```python
from build123d import *

# Parameters (mm, degrees)
F0_R     = 2.5
F1_DEPTH = 25
F3_R     = 15
F5_T     = -1


with BuildPart() as f1:
    # F0 (on Top) → F1 (new body)
    with BuildSketch(Plane.XY):
        Circle(F0_R)
    extrude(amount=F1_DEPTH)

    # F3 (on offset) → F4 section 0
    with BuildSketch(Plane.XY.offset(-20)):
        Circle(F3_R)
    # F0 (on Top) → F4 section 1
    with BuildSketch(Plane.XY):
        Circle(F0_R)
    loft()

    # F5
    f5_openings = [f1.faces().sort_by_distance(p)[0] for p in [
        (0, 0, 25),
        (0, 0, -20),
    ]]
    offset(amount=F5_T, openings=f5_openings, kind=Kind.INTERSECTION)


solid = f1.part
```
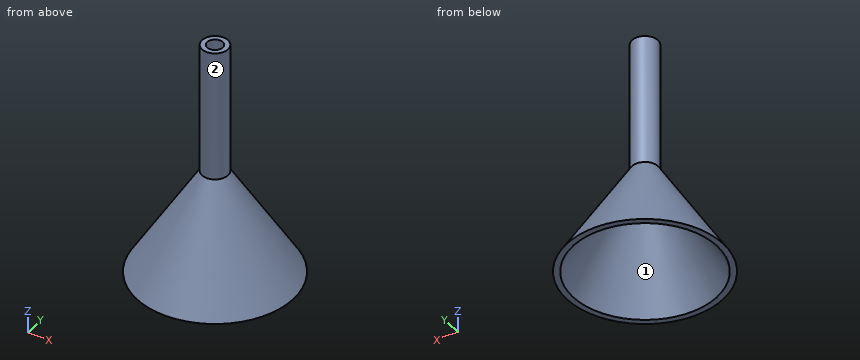
The listing builds one solid part. Answer for the finished solid, in the listing's coordinates (mm). Face numbers are marked on the shaded views. Round coordinates to 2 decimals unless told otherwise and drop trailing zeros. Write each loop counter-clockwise with the first axis right and the second up, starting at its lowest first coordinate (ties: lowest second). Pieces come first, ordered by that corner, then holes. Notation, with made-up numbers: (72.25, 54) -> (111.25, 54) arc R18 cw to (111.25, 72) -> close; hole circle Ø1 at (30.25, 45.5). An arc over 180 degrees is marked (long way). Answer as a JSON object with one key per item and string values. Group by question number.
Q1. Section A-A (x = 0) is taken. Write down the section's boundary in (y, z), plus the area to 3 significant figures.
Q2. Straight lines are drawn through the part: line 1 along Y through (x, z) = (0, 15.25); line 2 along Y through (x, z) = (-1.5, -12); line 3 along X through (y, z) = (-1, 3). For each, find the intervals that lie inside material, in ascending order.
Q3. Determine the mould class of the marked faces 1 and 2 for opening direction X: pulls with the +X half, pulls with the -X half, needs draft (parallel to the pull), parting line crosses it, or undercut.
Q4. Each of these flat-tipped pins is pushed along its axis until it touches: pin 1 Ø10 at (x, z) = (9, 9.5) entering from +Y; pin 2 Ø12 at (y, z) = (3.5, 0) entering from +X; pin 3 Ø10 at (x, z) = (-6, -12) entering from -Y; pin 4 Ø12 at (x, y) = (3, -5.5) entering from -Z. Where does it stop, or does it pass through?
Check values:
{
 "1": {"outline": "(-15, -20) -> (-13.82, -20) -> (-1.5, -0.29) -> (-1.5, 25) -> (-2.5, 25) -> (-2.5, 0) -> close; (1.5, -0.29) -> (13.82, -20) -> (15, -20) -> (2.5, 0) -> (2.5, 25) -> (1.5, 25) -> close", "area": "97.1 mm^2"},
 "2": {"line 1": "-2.5 to -1.5, 1.5 to 2.5", "line 2": "-9.89 to -8.69, 8.69 to 9.89", "line 3": "-2.29 to -1.12, 1.12 to 2.29"},
 "3": {"face 1": "undercut", "face 2": "parting line crosses it"},
 "4": {"pin 1": "through", "pin 2": "x = 5.85", "pin 3": "y = -12.23", "pin 4": "z = -17.51"}
}
